Geometry: final body of the model. Coordinates: model frame, mm. A direction names the side the tool comes from. Give positions to 0.01 mm unless a question says otherwise; leave off trailing zeros. Order: outer loops, then holes, each group sorted by start corner. A loop starts at its lowest first (then second) coordinate and runs counter-clockwise, first axis right, second up. Notation, with made-up numbers: (-19, 65.25) -> (24, 65.25) arc R8 cw to (24, 79.25) -> close; hole circle Ø8 at (0, 43.25). An arc over 180 degrees is marked (long way). One line per item, written item: value. Start each with the question number.
```python
from build123d import *

# Parameters (mm, degrees)
SKETCH1_W           = 35
SKETCH1_H           = 25
BOSS_EXTRUDE1_DEPTH = 10
SKETCH2_W           = 23
SKETCH2_H           = 13
CUT_EXTRUDE1_DEPTH  = 16
CUT_EXTRUDE3_REACH  = 31.368
SKETCH4_W           = 35
SKETCH4_H           = 4.915686931
FILLET2_R           = 5
FILLET3_R           = 5
FILLET4_R           = 5
FILLET5_R           = 5
CUT_EXTRUDE4_REACH  = 29.636
SKETCH3_R           = 1


with BuildPart() as part:
    # Sketch1 → Boss-Extrude1 (new, symmetric)
    with BuildSketch(Plane.XY):
        Rectangle(SKETCH1_W, SKETCH1_H)
    extrude(amount=BOSS_EXTRUDE1_DEPTH, both=True)

    # Sketch2 → Cut-Extrude1 (cut)
    with BuildSketch(Plane.XY.offset(10)):
        Rectangle(SKETCH2_W, SKETCH2_H)
    extrude(amount=-CUT_EXTRUDE1_DEPTH, mode=Mode.SUBTRACT)

    # Sketch4 → Cut-Extrude3 (cut, up to next)
    with BuildSketch(Plane.XY.offset(10), mode=Mode.PRIVATE) as cut_extrude3_sk1:
        with Locations((0, 10.042156535)):
            Rectangle(SKETCH4_W, SKETCH4_H)
    cut_extrude3_tool1 = extrude(cut_extrude3_sk1.sketch, amount=-CUT_EXTRUDE3_REACH, mode=Mode.PRIVATE) & part.part
    # Sketch4 → Cut-Extrude3 (cut, up to next)
    with BuildSketch(Plane.XY.offset(10), mode=Mode.PRIVATE) as cut_extrude3_sk2:
        with Locations((0, -10.042156535)):
            Rectangle(SKETCH4_W, SKETCH4_H)
    cut_extrude3_tool2 = extrude(cut_extrude3_sk2.sketch, amount=-CUT_EXTRUDE3_REACH, mode=Mode.PRIVATE) & part.part
    add(cut_extrude3_tool1.solids().sort_by_distance((0, 10.042157, 10))[0], mode=Mode.SUBTRACT)
    add(cut_extrude3_tool2.solids().sort_by_distance((0, -10.042157, 10))[0], mode=Mode.SUBTRACT)

    # Fillet2
    fillet2_edges = [part.edges().sort_by_distance(p)[0] for p in [
        (17.5, -7.584313069, 0),
    ]]
    fillet(fillet2_edges, radius=FILLET2_R)

    # Fillet3
    fillet3_edges = [part.edges().sort_by_distance(p)[0] for p in [
        (17.5, 7.584313069, 0),
    ]]
    fillet(fillet3_edges, radius=FILLET3_R)

    # Fillet4
    fillet4_edges = [part.edges().sort_by_distance(p)[0] for p in [
        (-17.5, 7.584313069, 0),
    ]]
    fillet(fillet4_edges, radius=FILLET4_R)

    # Fillet5
    fillet5_edges = [part.edges().sort_by_distance(p)[0] for p in [
        (-17.5, -7.584313069, 0),
    ]]
    fillet(fillet5_edges, radius=FILLET5_R)

    # Sketch3 → Cut-Extrude4 (cut, up to next)
    with BuildSketch(Plane.XY.offset(10), mode=Mode.PRIVATE) as cut_extrude4_sk1:
        with Locations((-13.9, 0)):
            Circle(SKETCH3_R)
    cut_extrude4_tool1 = extrude(cut_extrude4_sk1.sketch, amount=-CUT_EXTRUDE4_REACH, mode=Mode.PRIVATE) & part.part
    # Sketch3 → Cut-Extrude4 (cut, up to next)
    with BuildSketch(Plane.XY.offset(10), mode=Mode.PRIVATE) as cut_extrude4_sk2:
        with Locations(Location((13.9, 0, 0), (0, 0, 180))):
            Circle(SKETCH3_R)
    cut_extrude4_tool2 = extrude(cut_extrude4_sk2.sketch, amount=-CUT_EXTRUDE4_REACH, mode=Mode.PRIVATE) & part.part
    add(cut_extrude4_tool1.solids().sort_by_distance((-13.9, 0, 10))[0], mode=Mode.SUBTRACT)
    add(cut_extrude4_tool2.solids().sort_by_distance((13.9, 0, 10))[0], mode=Mode.SUBTRACT)


solid = part.part
```
1. Material intervals for L1, parallel to Y at x = 1.5, z = -5.5; L2, parallel to X at y = 2.5, z = 8.75; L3, parallel to X at y = -0.5, z = -6.5, sorted ascending. Write a range as [from, to].
2. Cut plane B-B, the plane y = 0. Return loops of the section in (x, z), then the cut area to 3 significant figures.
3. Draft query along X for faces 1 (the flat face through (11.5, 0, 2)), 2 (the cylindrical face through (-12.976, -0.383, 0.14)), 3 (the flat face through (0, -7, 10)), 4 (the flat face through (17.5, 0, 0)). Return one class per face: pulls with the +X half, pulls with the -X half, needs draft (parallel to the pull), parting line crosses it, or undercut.
4. Cut plane C-C, the plane x = 13.9. Return loops of the section in (y, z).
5. Cut plane A-A, the plane z = 3.75. Return loops of the section in (x, y), then the cut area to 3 significant figures.
6. Access query for faces 5 (the flat face through (0, 6.5, 2)), 6 (the cylindrical face through (16.074, 6.081, -0.14)). Directions: +Z, -Z, +X, -X, +Y, -Y. A direction counts if a zero-diameter tool reaches every point of the face in a straight line with its end or side. Return the directions, or none.
7. Cut plane D-D, the plane z = -7. Return loops of the section in (x, y).
8. Pin query (flat end, axial travel): P1, Ø1.6, axis at x = 13.9, y = 0, coming from the +Z side (1 decimal). Return the tip coordinate at first contact, or that it passes through.
Answers follow:
1. L1: y = [-7.58, -6.5], [6.5, 7.58]
1. L2: x = [-17.5, -11.5], [11.5, 17.5]
1. L3: x = [-17.5, -14.77], [-13.03, 13.03], [14.77, 17.5]
2. outline: (-17.5, -10) -> (-14.9, -10) -> (-14.9, 10) -> (-17.5, 10) -> close; (-12.9, -10) -> (12.9, -10) -> (12.9, 10) -> (11.5, 10) -> (11.5, -6) -> (-11.5, -6) -> (-11.5, 10) -> (-12.9, 10) -> close; (14.9, -10) -> (17.5, -10) -> (17.5, 10) -> (14.9, 10) -> close
2. area: 252 mm²
3. face 1: undercut
3. face 2: undercut
3. face 3: needs draft
3. face 4: pulls with the +X half
4. outline: (-7.38, -10) -> (-1, -10) -> (-1, 10) -> (-7.38, 10) -> close; (1, -10) -> (7.38, -10) -> (7.38, 10) -> (1, 10) -> close
5. outline: (-17.5, -2.58) arc R5 ccw to (-12.5, -7.58) -> (12.5, -7.58) arc R5 ccw to (17.5, -2.58) -> (17.5, 2.58) arc R5 ccw to (12.5, 7.58) -> (-12.5, 7.58) arc R5 ccw to (-17.5, 2.58) -> close; hole circle Ø2 at (-13.9, 0); hole (-11.5, -6.5) -> (11.5, -6.5) -> (11.5, 6.5) -> (-11.5, 6.5) -> close; hole circle Ø2 at (13.9, 0)
5. area: 204 mm²
6. face 5: +Z
6. face 6: +Z, -Z, +X, +Y
7. outline: (-17.5, -2.58) arc R5 ccw to (-12.5, -7.58) -> (12.5, -7.58) arc R5 ccw to (17.5, -2.58) -> (17.5, 2.58) arc R5 ccw to (12.5, 7.58) -> (-12.5, 7.58) arc R5 ccw to (-17.5, 2.58) -> close; hole circle Ø2 at (-13.9, 0); hole circle Ø2 at (13.9, 0)
8. P1: passes through
